The listing builds one solid part. Answer for the finished solid, in the listing's coordinates (mm). Face numbers are marked on the shaded views. Coordinates: 2 decimals unless noted, no trailing zeros. Write each loop counter-clockwise with the first axis right and the second up, starting at its lowest first coordinate (ties: lowest second). Pieces come first, ordered by that corner, then holes.
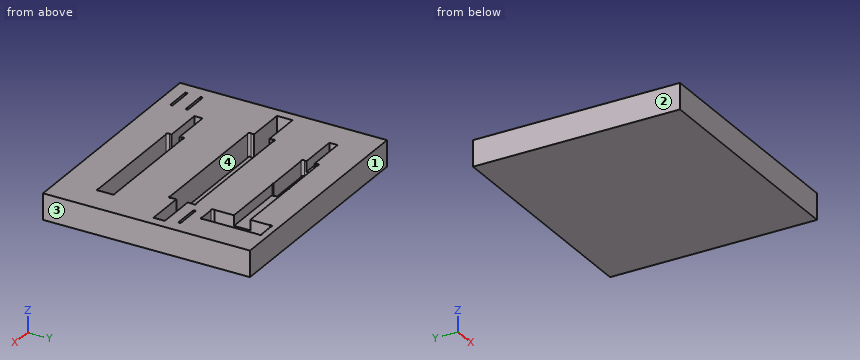
from build123d import *

# Parameters (mm, degrees)
F0_W      = 114.3
F0_H      = 76.2
F1_DEPTH  = 12.7
F3_DEPTH  = 11.43
F4_W      = 12.7
F4_H      = 1.143
F5_DEPTH  = 11.43
F8_DEPTH  = 11.43
F9_R      = 0.75
F10_DEPTH = 11.43
F11_W     = 114.3
F11_H     = 24.9555
F12_DEPTH = 12.7
F14_DEPTH = 11.43
F16_DEPTH = 5.08
F18_W     = 25.4
F18_H     = 8.001
F19_DEPTH = 2.54
F21_R     = 0.75
F22_DEPTH = 7.62
F23_R     = 0.75
F24_DEPTH = 11.43


with BuildPart() as f1:
    # F0 (on Top) → F1 (new body)
    with BuildSketch(Plane.XY):
        with Locations((-57.15, -38.1)):
            Rectangle(F0_W, F0_H)
    extrude(amount=F1_DEPTH)

    # F2 (on face) → F3 (cut)
    with BuildSketch(Plane.XY.offset(12.7)):
        Polygon((-90.4875, -18.415), (-109.5375, -18.415), (-109.5375, -26.035), (-90.4875, -26.035), (-90.4875, -28.575), (-23.8125, -28.575), (-23.8125, -25.019), (-4.7625, -25.019), (-4.7625, -19.431), (-23.8125, -19.431), (-23.8125, -15.875), (-90.4875, -15.875), align=None)
    extrude(amount=-F3_DEPTH, mode=Mode.SUBTRACT)

    # F4 (on face) → F5 (cut)
    with BuildSketch(Plane.XY.offset(12.7)):
        with Locations((-12.7, -13.2715)):
            Rectangle(F4_W, F4_H)
        with Locations((-101.6, -69.2785)):
            Rectangle(F4_W, F4_H)
        with Locations((-101.6, -61.7855)):
            Rectangle(F4_W, F4_H)
    extrude(amount=-F5_DEPTH, mode=Mode.SUBTRACT)

    # F7 (on face) → F8 (cut)
    with BuildSketch(Plane.XY.offset(12.7)):
        Polygon((-91.7575, -55.975), (-72.7075, -55.975), (-72.7075, -58.039), (-13.97, -58.039), (-13.97, -49.911), (-72.7075, -49.911), (-72.7075, -51.975), (-91.7575, -51.975), align=None)
    extrude(amount=-F8_DEPTH, mode=Mode.SUBTRACT)

    # F9 (on face) → F10 (cut)
    with BuildSketch(Plane.XY.offset(12.7)):
        with Locations((-89.9571699141, -16.4053300859)):
            Circle(F9_R)
        with Locations((-89.9571699141, -28.0446699141)):
            Circle(F9_R)
        with Locations((-24.3428300859, -28.0446699141)):
            Circle(F9_R)
        with Locations((-24.3428300859, -16.4053300859)):
            Circle(F9_R)
        with Locations((-14.5003300859, -50.4413300859)):
            Circle(F9_R)
        with Locations((-14.5003300859, -57.5086699141)):
            Circle(F9_R)
        with Locations((-72.1771699141, -50.4413300859)):
            Circle(F9_R)
        with Locations((-72.1771699141, -57.5086699141)):
            Circle(F9_R)
    extrude(amount=-F10_DEPTH, mode=Mode.SUBTRACT)

    # F11 (on face) → F12 (join)
    with BuildSketch(Plane.XY.offset(12.7)):
        with Locations((-57.15, 12.47775)):
            Rectangle(F11_W, F11_H)
    extrude(amount=-F12_DEPTH)

    # F13 (on face) → F14 (cut)
    with BuildSketch(Plane.XY.offset(12.7)):
        Polygon((-14.2875, 21.7805), (-23.8125, 21.7805), (-23.8125, 11.176), (-23.8125, 3.175), (-23.8125, -7.4295), (-14.2875, -7.4295), align=None)
    extrude(amount=-F14_DEPTH, mode=Mode.SUBTRACT)

    # F15 (on face) → F16 (cut)
    with BuildSketch(Plane.XY.offset(12.7)):
        Polygon((-23.8125, 11.176), (-80.9625, 11.176), (-80.9625, 9.1755), (-100.0125, 9.1755), (-100.0125, 5.1755), (-80.9625, 5.1755), (-80.9625, 3.175), (-23.8125, 3.175), align=None)
    extrude(amount=-F16_DEPTH, mode=Mode.SUBTRACT)

    # F18 (on 3pt) → F19 (cut)
    with BuildSketch(Plane.XY.offset(7.62)):
        with Locations((-68.2625, 7.1755)):
            Rectangle(F18_W, F18_H)
    extrude(amount=-F19_DEPTH, mode=Mode.SUBTRACT)

    # F21 (on face) → F22 (cut)
    with BuildSketch(Plane.XY.offset(12.7)):
        with Locations((-56.0928300859, 10.6456699141)):
            Circle(F21_R)
        with Locations((-56.0928300859, 3.7053300859)):
            Circle(F21_R)
        with Locations((-80.4321699141, 3.7053300859)):
            Circle(F21_R)
        with Locations((-80.4321699141, 10.6456699141)):
            Circle(F21_R)
    extrude(amount=-F22_DEPTH, mode=Mode.SUBTRACT)

    # F23 (on face) → F24 (cut)
    with BuildSketch(Plane.XY.offset(12.7)):
        with Locations((-23.2821699141, -6.8991699141)):
            Circle(F23_R)
        with Locations((-14.8178300859, -6.8991699141)):
            Circle(F23_R)
        with Locations((-23.2821699141, 21.2501699141)):
            Circle(F23_R)
        with Locations((-14.8178300859, 21.2501699141)):
            Circle(F23_R)
    extrude(amount=-F24_DEPTH, mode=Mode.SUBTRACT)


solid = f1.part
Q1. The part is cut by section B-B, the plane y = 16. Write down the section's boundary in (x, z).
Answers below:
outline: (-114.3, 0) - (0, 0) - (0, 12.7) - (-14.29, 12.7) - (-14.29, 1.27) - (-23.81, 1.27) - (-23.81, 12.7) - (-114.3, 12.7) - close
Q2. The part is cut by section D-D, the plane x = -84. Write down the section's boundary in (y, z) (1 decimal), then the cut area to 3 significant figures.
Answers below:
outline: (-76.2, 0) - (25, 0) - (25, 12.7) - (9.2, 12.7) - (9.2, 7.6) - (5.2, 7.6) - (5.2, 12.7) - (-15.9, 12.7) - (-15.9, 1.3) - (-28.6, 1.3) - (-28.6, 12.7) - (-52, 12.7) - (-52, 1.3) - (-56, 1.3) - (-56, 12.7) - (-76.2, 12.7) - close
area: 1,070 mm2
Q3. The part is cut by section C-C, the plane z = 9.5. State how many separate pieces and enclosed holes the cut face has, then the cut area to 3 significant figures.
Answers below:
separate pieces: 1
enclosed holes: 6
area: 9,050 mm2
Q4. The part is cut by section A-A, the plane x = -43. Write down the section's boundary in (y, z) (1 decimal), then the cut area to 3 significant figures.
Answers below:
outline: (-76.2, 0) - (25, 0) - (25, 12.7) - (11.2, 12.7) - (11.2, 7.6) - (3.2, 7.6) - (3.2, 12.7) - (-15.9, 12.7) - (-15.9, 1.3) - (-28.6, 1.3) - (-28.6, 12.7) - (-49.9, 12.7) - (-49.9, 1.3) - (-58, 1.3) - (-58, 12.7) - (-76.2, 12.7) - close
area: 1,010 mm2
Q5. Find the intervals of material crossed by probe 1 along Y at (x, z) = (-69, 6) (1 decimal); probe 2 along Y at (x, z) = (-12.5, 7.5); probe 3 along X at (y, z) = (-3.5, 6.75), in increasing order.
Answers below:
probe 1: y = -76.2 to -58, -49.9 to -28.6, -15.9 to 3.2, 11.2 to 25
probe 2: y = -76.2 to -25.02, -19.43 to -13.84, -12.7 to 24.96
probe 3: x = -114.3 to -23.81, -14.29 to 0
Q6. Determine the mould class of the marked faces 1, 2, 3 and 4 for opening direction X: released by +X, released by -X, zero draft, split by the parting line, or undercut.
Answers below:
face 1: zero draft
face 2: released by -X
face 3: released by +X
face 4: undercut
Q7. Given pin 1 (2.5 mm diameter, centred on x = -66.5, y = -52.5, fed in from +Z); pin 2 (3 mm diameter, centred on x = -88.5, y = 7, fed in from +Z), each flat-ended and moving along its own axis, determine where each tip first touches the part or whether it passes through.
Answers below:
pin 1: stops at z = 1.27
pin 2: stops at z = 7.62
